Study the drawing (mm; zero at the part's minimum x, y, z) and answer. A direction names the side the tool comes from. Give positions to 0.01 mm unless a question says otherwise; leave off trailing zeros. Order: outer loops, then holes, each group sorted by start corner. A loop starts at its lowest first (then second) coordinate and runs counter-clockwise, first axis right, second up.
Item 1: Find the intervals of material crossed by line 1 along Z through (x, y) = (15, 92.75); line 2 along X through (y, z) = (28.5, 15.25); line 3 along Z through (x, y) = (15, 96.75), in increasing order.
Item 2: A cutting plane is placed at C-C (y = 55.5). Write down the section's boundary in (x, z).
Item 3: A cutting plane is placed at B-B (z = 15). Write down the section's boundary in (x, y), plus the area to 3 significant figures.
Item 4: Given pin 1 Ø5 at (x, y) = (15.5, 32) entering from +Z; pin 2 Ø2 at (y, z) = (32.5, 25.5) entering from +X; pin 3 Ø3 at (y, z) = (68.5, 22) entering from +X; pin 4 Ø12 at (y, z) = (82, 6.5) entering from +X, each flat-ended and moving along its own axis, determine where each tip first touches the part or whether it passes through.
Item 5: Which of the six approach directions +Z, -Z, +X, -X, +Y, -Y give full straight-line access (tool end or side, diameter ignored) to the marked faces 1 and 2?
Item 6: A cutting plane is placed at A-A (x = 15). Write down the section's boundary in (y, z), plus the area to 3 significant figures.
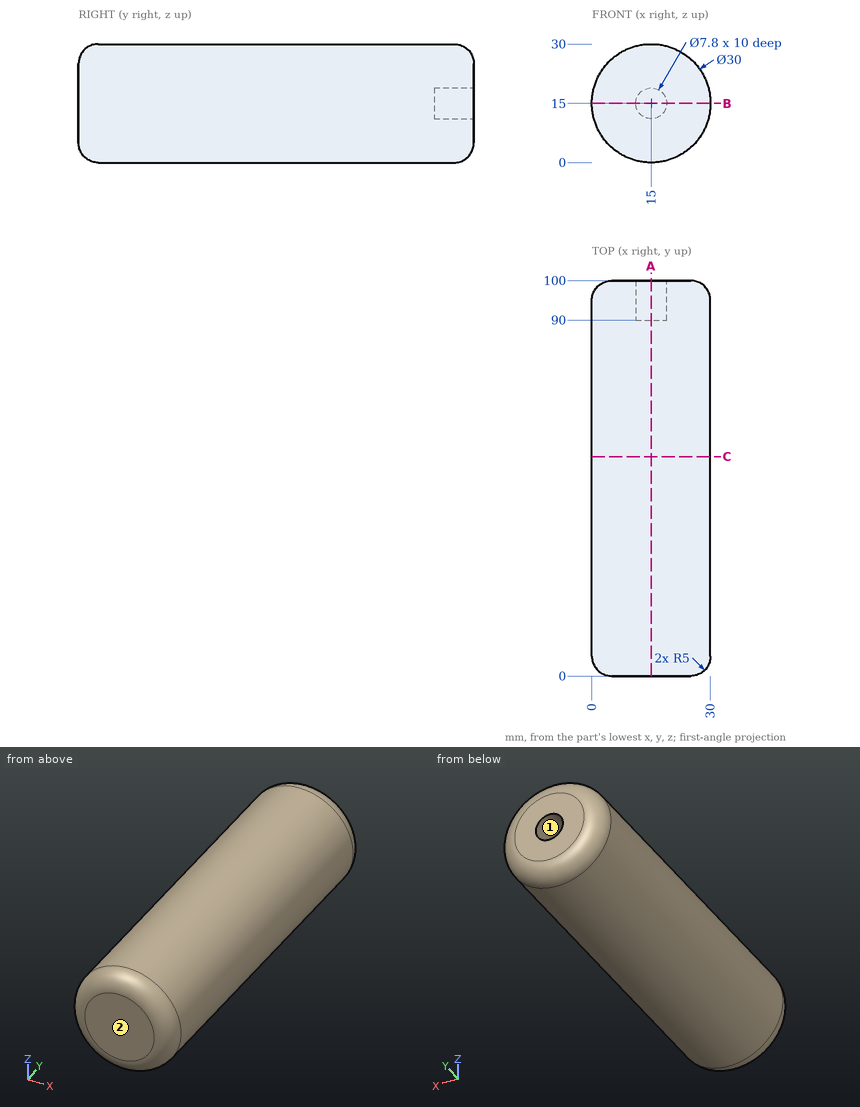
Response values:
1. line 1: z = 0 to 11.1, 18.9 to 30
1. line 2: x = 0 to 30
1. line 3: z = 0.32 to 11.1, 18.9 to 29.68
2. outline: circle Ø30 at (15, 15)
3. outline: (0, 5) arc R5 ccw to (5, 0) - (25, 0) arc R5 ccw to (30, 5) - (30, 95) arc R5 ccw to (25, 100) - (18.9, 100) - (18.9, 90) - (11.1, 90) - (11.1, 100) - (5, 100) arc R5 ccw to (0, 95) - close
3. area: 2,900 mm2
4. pin 1: stops at z = 30
4. pin 2: stops at x = 26.61
4. pin 3: stops at x = 28.96
4. pin 4: stops at x = 29.79
5. face 1: +Y
5. face 2: +Z, -Z, +X, -X, -Y
6. outline: (0, 5) arc R5 ccw to (5, 0) - (95, 0) arc R5 ccw to (100, 5) - (100, 11.1) - (90, 11.1) - (90, 18.9) - (100, 18.9) - (100, 25) arc R5 ccw to (95, 30) - (5, 30) arc R5 ccw to (0, 25) - close
6. area: 2,900 mm2
